Drawing for the job (mm, zero at the part's lowest x, y, z). Round coordinates to 2 decimals unless told otherwise and drop trailing zeros. Loops run counter-clockwise (first coordinate to the right, second up) from the corner with the lowest first, then second, coordinate; pieces in that order, holes last. Notation, with made-up numbers: (-32.75, -19.75) - (-2.75, -19.75) arc R22 cw to (-2.75, -2.75) - close; hole circle Ø7 at (48, -39.75). An arc over 180 degrees is marked (long way). Put each result on its own line as item: value.
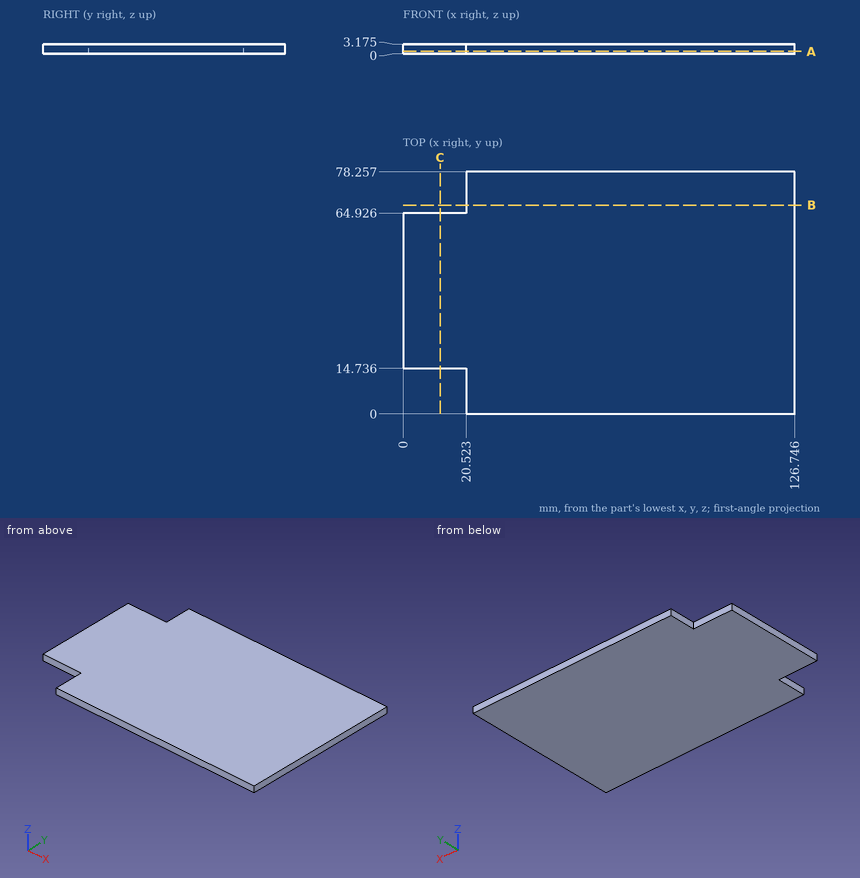
1. Probe line 1 along X through (y, z) = (13, 1.3). List the from-to ranges inside material, lowest first. Write a range as [from, to].
A:
line 1: x = [20.52, 126.75]
2. Pin check, flat tips, straight feed: P1, Ø1.6, axis at y = 5.5, z = 1, coming from the -X side; P2, Ø1, axis at x = 44.5, z = 2.5, coming from the -Y side. Stop position of each tip, or through.
A:
P1: stops at x = 20.52
P2: stops at y = 0
3. Band-saw the part on A-A (z = 0.75). List the corners of the cut face in (x, y), plus the area to 3 significant figures.
A:
outline: (0, 14.74) - (20.52, 14.74) - (20.52, 0) - (126.75, 0) - (126.75, 78.26) - (20.52, 78.26) - (20.52, 64.93) - (0, 64.93) - close
area: 9,340 mm²
4. Band-saw the part on C-C (x = 12). List the corners of the cut face in (y, z) (1 decimal), plus the area to 3 significant figures.
A:
outline: (14.7, 0) - (64.9, 0) - (64.9, 3.2) - (14.7, 3.2) - close
area: 159 mm²
5. Band-saw the part on B-B (y = 67.5). List the corners of the cut face in (x, z) (1 decimal).
A:
outline: (20.5, 0) - (126.7, 0) - (126.7, 3.2) - (20.5, 3.2) - close
